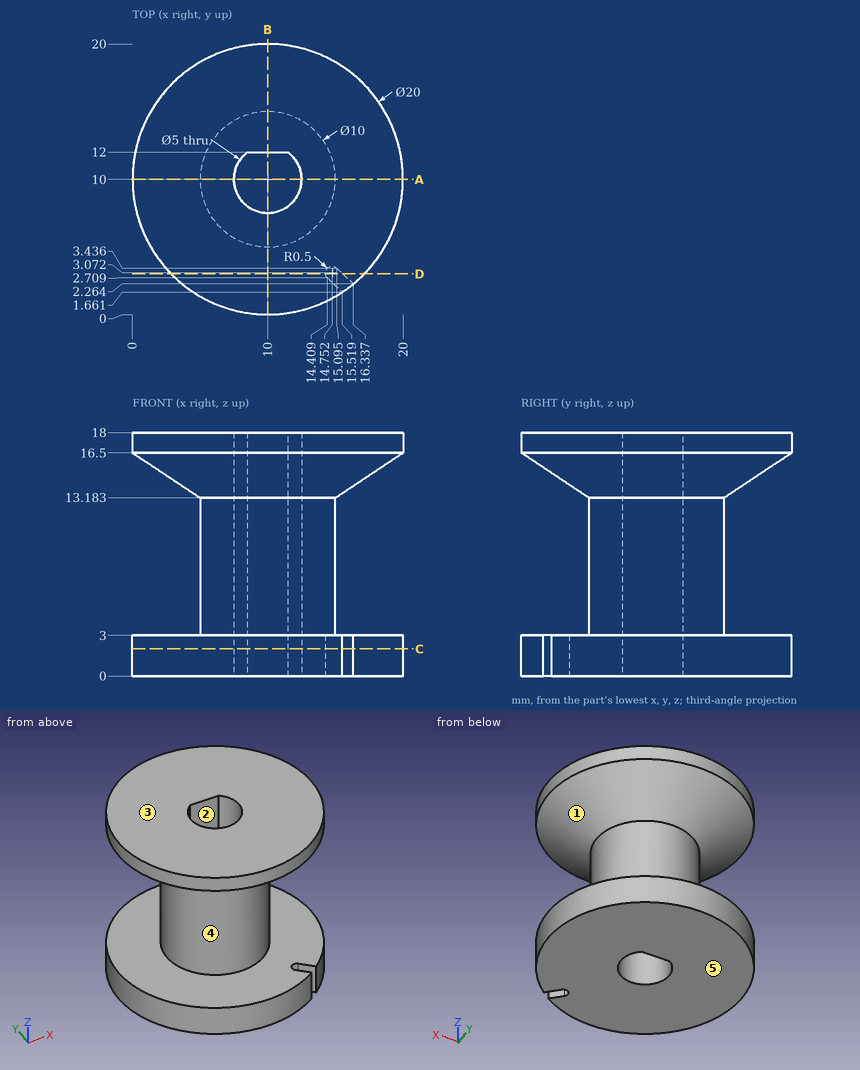
The figure shows three views and two pictorial views of one solid part (mm, origin at its lowest corner). Answer the questions. A direction names the side the tool comes from. Round coordinates to 2 decimals unless told otherwise and drop trailing zeros. Order: outer loops, then holes, each group sorted by start corner. A loop starts at its lowest first (then second) coordinate and runs counter-clockwise, first axis right, second up. Notation, with made-up numbers: (35.5, 14) -> (72.5, 14) arc R22 cw to (72.5, 51) -> close; hole circle Ø8 at (-22, -37.75). An arc over 180 degrees is marked (long way). One line per item, written item: value.
Item 1: Find section B-B, the plane x = 10. Give the vertices of the cut face in (y, z).
Taken from the geometry:
outline: (0, 0) -> (7.5, 0) -> (7.5, 18) -> (0, 18) -> (0, 16.5) -> (5, 13.18) -> (5, 3) -> (0, 3) -> close; (12, 0) -> (20, 0) -> (20, 3) -> (15, 3) -> (15, 13.18) -> (20, 16.5) -> (20, 18) -> (12, 18) -> close
Item 2: For the marked faces 1 and 2, determine the directions among +Z, -Z, +X, -X, +Y, -Y from which every point of the face is accessible in a straight line to the end or side of a thin tool.
Taken from the geometry:
face 1: none
face 2: +Z, -Z
Item 3: Find section D-D, the plane y = 3. State how many separate pieces and enclosed holes the cut face has.
Taken from the geometry:
separate pieces: 3
enclosed holes: 0
Item 4: Given P1, Ø8, axis at y = 13.5, z = 11.5, coming from the -X side (1 decimal); P2, Ø2, axis at x = 14, z = 8, coming from the +Y side; P3, Ø1, axis at y = 13, z = 5.5, coming from the -X side, each flat-ended and moving along its own axis, determine where each tip first touches the part or whether it passes through.
Taken from the geometry:
P1: stops at x = 2.1
P2: stops at y = 14
P3: stops at x = 5.67
Item 5: Find section C-C, the plane z = 2. Give the vertices of the cut face in (x, y) (1 decimal).
Taken from the geometry:
outline: (14.4, 2.7) arc R0.5 cw to (15.1, 3.4) -> (16.3, 2.3) arc R10 ccw (long way) to (15.5, 1.7) -> close; hole (8.5, 12) arc R2.5 ccw (long way) to (11.5, 12) -> close
Item 6: For a pull along Z with two mould halves and no side action, classify the marked faces 3, 4 and 5 as released by +Z, released by -Z, zero draft, split by the parting line, or undercut.
Taken from the geometry:
face 3: released by +Z
face 4: undercut
face 5: released by -Z
Item 7: Straight lines are drawn through the part: L1, parallel to X at y = 10, z = 8.75; L2, parallel to Y at x = 10, z = 6.5; L3, parallel to Z at x = 4.25, y = 13.75. For each, find the intervals that lie inside material, in ascending order.
Taken from the geometry:
L1: x = 5 to 7.5, 12.5 to 15
L2: y = 5 to 7.5, 12 to 15
L3: z = 0 to 3, 14.42 to 18
Item 8: Find section A-A, the plane y = 10. Give the vertices of the cut face in (x, z).
Taken from the geometry:
outline: (0, 0) -> (7.5, 0) -> (7.5, 18) -> (0, 18) -> (0, 16.5) -> (5, 13.18) -> (5, 3) -> (0, 3) -> close; (12.5, 0) -> (20, 0) -> (20, 3) -> (15, 3) -> (15, 13.18) -> (20, 16.5) -> (20, 18) -> (12.5, 18) -> close
